Build history of the part. All positions in model axes, mm. A direction names the side the tool comes from. Round coordinates to 2 decimals unless told otherwise and drop trailing zeros. Loops run counter-clockwise (first coordinate to the right, second up) from the corner with the lowest first, then second, coordinate; pieces in that order, holes last. Notation, with made-up numbers: (-18, 11.25) - (16, 11.25) arc R36 cw to (16, 46.25) - close; hole circle Ø6 at (61, -35). An arc over 180 degrees is marked (long way). One line per question, with ' | ' between items. Start each with the question number.
from build123d import *

# Parameters (mm, degrees)
BOSS_EXTRUDE3_DEPTH = 11.049
SKETCH2_W           = 9.652
SKETCH2_H           = 6.604
SKETCH2_W_2         = 6.604
CUT_EXTRUDE1_DEPTH  = 8.255
SKETCH5_W           = 3.429
SKETCH5_H           = 5.08
BOSS_EXTRUDE4_DEPTH = 5.08
SKETCH6_W           = 9.652
SKETCH6_H           = 1.524
BOSS_EXTRUDE5_DEPTH = 5.08
CUT_EXTRUDE3_DEPTH  = 5.08
CUT_EXTRUDE4_START  = -0.0508
CUT_EXTRUDE4_DEPTH  = 0.0508
CUT_EXTRUDE5_DEPTH  = 0.0508


# Read off the part's stored shape, not the designer's step: Cut-Extrude4
with BuildPart() as part:
    # Sketch1 → Boss-Extrude3 (new body)
    with BuildSketch(Plane(origin=(0, 0, 0), x_dir=(1, 0, 0), z_dir=(0, 1, 0))):
        with BuildLine():
            ThreePointArc((-12.7635, 3.302), (-16.0655, 0), (-12.7635, -3.302))
            Line((-12.7635, -3.302), (-12.7635, -1.651))
            ThreePointArc((-12.7635, -1.651), (-14.4145, 0), (-12.7635, 1.651))
            Line((-12.7635, 1.651), (-12.7635, 3.302))
        make_face()
        with BuildLine():
            Line((-12.7635, -1.651), (-12.7635, -3.302))
            ThreePointArc((-12.7635, -3.302), (-10.428633409, -2.334866591), (-9.4615, 0))
            ThreePointArc((-9.4615, 0), (-10.428633409, 2.334866591), (-12.7635, 3.302))
            Line((-12.7635, 3.302), (-12.7635, 1.651))
            ThreePointArc((-12.7635, 1.651), (-11.596066704, 1.167433296), (-11.1125, 0))
            ThreePointArc((-11.1125, 0), (-11.596066704, -1.167433296), (-12.7635, -1.651))
        make_face()
        with BuildLine():
            Line((-12.7635, -3.302), (12.7635, -3.302))
            ThreePointArc((12.7635, -3.302), (9.4615, 0), (12.7635, 3.302))
            Line((12.7635, 3.302), (-12.7635, 3.302))
            ThreePointArc((-12.7635, 3.302), (-10.428633409, 2.334866591), (-9.4615, 0))
            ThreePointArc((-9.4615, 0), (-10.428633409, -2.334866591), (-12.7635, -3.302))
        make_face()
        with BuildLine():
            ThreePointArc((12.7635, 3.302), (9.4615, 0), (12.7635, -3.302))
            Line((12.7635, -3.302), (12.7635, -1.651))
            ThreePointArc((12.7635, -1.651), (11.1125, 0), (12.7635, 1.651))
            Line((12.7635, 1.651), (12.7635, 3.302))
        make_face()
        with BuildLine():
            Line((12.7635, -1.651), (12.7635, -3.302))
            ThreePointArc((12.7635, -3.302), (15.098366591, -2.334866591), (16.0655, 0))
            ThreePointArc((16.0655, 0), (15.098366591, 2.334866591), (12.7635, 3.302))
            Line((12.7635, 3.302), (12.7635, 1.651))
            ThreePointArc((12.7635, 1.651), (13.930933296, 1.167433296), (14.4145, 0))
            ThreePointArc((14.4145, 0), (13.930933296, -1.167433296), (12.7635, -1.651))
        make_face()
    extrude(amount=BOSS_EXTRUDE3_DEPTH)

    # Sketch2 → Cut-Extrude1 (cut)
    with BuildSketch(Plane(origin=(0, 11.049, 0), x_dir=(1, 0, 0), z_dir=(0, 1, 0))):
        Rectangle(SKETCH2_W, SKETCH2_H)
        with Locations((12.7635, 0)):
            Rectangle(SKETCH2_W_2, SKETCH2_H)
        with Locations((-12.7635, 0)):
            Rectangle(SKETCH2_W_2, SKETCH2_H)
    extrude(amount=-CUT_EXTRUDE1_DEPTH, mode=Mode.SUBTRACT)

    # Sketch5 → Boss-Extrude4 (add)
    with BuildSketch(Plane.XZ):
        with Locations((6.5405, 0.056957201)):
            Rectangle(SKETCH5_W, SKETCH5_H)
        with Locations((-6.5405, 0.056957201)):
            Rectangle(SKETCH5_W, SKETCH5_H)
    extrude(amount=BOSS_EXTRUDE4_DEPTH)

    # Sketch6 → Boss-Extrude5 (add)
    with BuildSketch(Plane.XZ):
        Rectangle(SKETCH6_W, SKETCH6_H)
    extrude(amount=BOSS_EXTRUDE5_DEPTH)

    # Sketch7 → Cut-Extrude3 (cut)
    with BuildSketch(Plane.XY.offset(0.762)):
        with BuildLine():
            ThreePointArc((-4.826, -5.08), (-0.756934481, -11.57255329), (5.052785714, -6.576785714))
            ThreePointArc((5.052785714, -6.576785714), (4.995767575, -5.819851233), (4.826, -5.08))
            Line((4.826, -5.08), (-4.826, -5.08))
        make_face()
        with BuildLine():
            Line((-4.826, -5.08), (4.826, -5.08))
            ThreePointArc((4.826, -5.08), (2.997307625, -2.50901108), (0, -1.524))
            ThreePointArc((0, -1.524), (-2.997307625, -2.50901108), (-4.826, -5.08))
        make_face()
    extrude(amount=-CUT_EXTRUDE3_DEPTH, mode=Mode.SUBTRACT)

    # Cut-Extrude4 outline → Cut-Extrude4 (cut)
    with BuildSketch(Plane(origin=(0, 11.049, 0), x_dir=(1, 0, 0), z_dir=(0, 1, 0)).offset(CUT_EXTRUDE4_START)):
        with BuildLine():
            Line((6.125651291, -1.107505234), (5.764715133, -1.322388012))
            add(Edge.make_bspline(
                [(5.764715133, -1.322388012), (5.795848726, -1.396544386), (5.855526361, -1.499286266), (5.978159662, -1.669974458), (6.05114933, -1.775594986), (6.148137968, -1.884253365), (6.256046735, -1.979672728), (6.372017343, -2.072531851), (6.478000588, -2.125037114), (6.583983834, -2.177542378), (6.687715089, -2.205891048), (6.772837481, -2.228601824), (6.855428053, -2.259126551), (6.956720766, -2.259126551), (7.082059087, -2.259126551), (7.202566961, -2.259126551), (7.355228923, -2.239958049), (7.545854824, -2.189191034), (7.64564176, -2.137070791), (7.756302185, -2.074391176), (7.861852333, -1.998233742), (7.956762183, -1.91923746), (8.138419792, -1.696975289), (8.222600111, -1.522442374), (8.284179667, -1.341062147), (8.308803358, -1.188392086), (8.308803358, -1.045195403), (8.257662319, -0.813306269), (8.216986985, -0.673773492), (8.132229192, -0.510521819), (7.993166094, -0.321750968), (7.909998502, -0.224416829), (7.802295587, -0.121226034), (7.6621337, 0.004412918), (7.5566666, 0.088832099), (7.079288797, 0.442114266), (6.827397054, 0.625925615), (6.758715893, 0.678132356), (6.698618911, 0.734864272), (6.648436244, 0.783693405), (6.615575385, 0.819143072), (6.575738864, 0.868399704), (6.535888686, 0.916871649), (6.495665853, 0.988895848), (6.455893708, 1.086814708), (6.435475968, 1.172671893), (6.422326559, 1.281945673), (6.441309585, 1.39829107), (6.467008859, 1.482949614), (6.517139065, 1.57939298), (6.576546974, 1.648262165), (6.660252521, 1.721257683), (6.76204807, 1.770361107), (6.850036001, 1.799422275), (6.919376094, 1.821827394), (7.000254698, 1.821827394), (7.060862271, 1.821827394), (7.158295762, 1.821827394), (7.245490979, 1.805342484), (7.330857485, 1.780448172), (7.394182968, 1.74575823), (7.422569964, 1.733524046), (7.454232705, 1.716179075), (7.490911825, 1.697072046), (7.514106284, 1.676478569), (7.564005826, 1.643675962), (7.656944095, 1.554409737), (7.739669602, 1.474435351), (7.776778642, 1.43169931), (7.842489762, 1.361666912), (7.905039475, 1.278267425)],
                knots=[0, 0, 0, 0, 0, 0, 0, 0, 0.015625, 0.03125, 0.046875, 0.0625, 0.078125, 0.09375, 0.109375, 0.125, 0.140625, 0.15625, 0.171875, 0.1875, 0.203125, 0.21875, 0.234375, 0.25, 0.265625, 0.28125, 0.296875, 0.3125, 0.328125, 0.34375, 0.359375, 0.375, 0.390625, 0.40625, 0.421875, 0.4375, 0.453125, 0.46875, 0.484375, 0.5, 0.515625, 0.53125, 0.546875, 0.5625, 0.578125, 0.59375, 0.609375, 0.625, 0.640625, 0.65625, 0.671875, 0.6875, 0.703125, 0.71875, 0.734375, 0.75, 0.765625, 0.78125, 0.796875, 0.8125, 0.828125, 0.84375, 0.859375, 0.875, 0.890625, 0.90625, 0.921875, 0.9375, 0.953125, 0.96875, 0.984375, 1, 1, 1, 1, 1, 1, 1, 1], degree=7))
            Line((7.905039475, 1.278267425), (8.253289165, 1.539455103))
            add(Edge.make_bspline(
                [(8.253289165, 1.539455103), (8.156895883, 1.66119447), (8.080596703, 1.752467641), (8.009921379, 1.822625174), (7.933726759, 1.919905891), (7.824588167, 2.017677373), (7.667478791, 2.113158926), (7.554717937, 2.174929753), (7.426668873, 2.21890102), (7.295363504, 2.247898039), (7.181818455, 2.267110724), (7.014103692, 2.267110724), (6.815864787, 2.237013824), (6.659136337, 2.182262131), (6.55037867, 2.129800369), (6.423181047, 2.050572345), (6.335021768, 1.976771869), (6.231051482, 1.855134106), (6.149145224, 1.716981286), (6.084448013, 1.567732126), (6.040533381, 1.421764923), (6.040533381, 1.293676397), (6.040533381, 1.143393573), (6.070495088, 0.985652762), (6.137396877, 0.821399612), (6.210558512, 0.692920171), (6.259072046, 0.646259485), (6.293158014, 0.580378426), (6.471822739, 0.420467618), (6.75149803, 0.193678775), (6.790287956, 0.170783169), (7.498283405, -0.384707414), (7.577864327, -0.459159137), (7.65987138, -0.544113603), (7.728973771, -0.621025877), (7.79510367, -0.718827072), (7.865584999, -0.866409444), (7.892864321, -0.947931981), (7.924722723, -1.016219237), (7.924722723, -1.066155835), (7.908904135, -1.168139886), (7.908904135, -1.225535848), (7.873403325, -1.31658975), (7.846091508, -1.386832441), (7.81374531, -1.446533535), (7.789405983, -1.495887306), (7.72836903, -1.555160993), (7.677947198, -1.604126212), (7.627570897, -1.65047546), (7.548458311, -1.699013274), (7.474880936, -1.729316994), (7.409037252, -1.764969223), (7.304160871, -1.794806682), (7.188897018, -1.818103802), (7.115683884, -1.818103802), (7.027185487, -1.818103802), (6.93589672, -1.818103802), (6.863229947, -1.796088084), (6.759400758, -1.765758188), (6.658680651, -1.706691455), (6.586423649, -1.661131989), (6.506706136, -1.594528182), (6.442547065, -1.533389449), (6.378433525, -1.469634745), (6.304296754, -1.382180872), (6.232995884, -1.281685995), (6.192311068, -1.220896958), (6.149245652, -1.146989207), (6.125651291, -1.107505234)],
                knots=[0, 0, 0, 0, 0, 0, 0, 0, 0.016129032, 0.032258065, 0.048387097, 0.064516129, 0.080645161, 0.096774194, 0.112903226, 0.129032258, 0.14516129, 0.161290323, 0.177419355, 0.193548387, 0.209677419, 0.225806452, 0.241935484, 0.258064516, 0.274193548, 0.290322581, 0.306451613, 0.322580645, 0.338709677, 0.35483871, 0.370967742, 0.387096774, 0.403225806, 0.419354839, 0.435483871, 0.451612903, 0.467741935, 0.483870968, 0.5, 0.516129032, 0.532258065, 0.548387097, 0.564516129, 0.580645161, 0.596774194, 0.612903226, 0.629032258, 0.64516129, 0.661290323, 0.677419355, 0.693548387, 0.709677419, 0.725806452, 0.741935484, 0.758064516, 0.774193548, 0.790322581, 0.806451613, 0.822580645, 0.838709677, 0.85483871, 0.870967742, 0.887096774, 0.903225806, 0.919354839, 0.935483871, 0.951612903, 0.967741935, 0.983870968, 1, 1, 1, 1, 1, 1, 1, 1], degree=7))
        make_face()
    extrude(amount=CUT_EXTRUDE4_DEPTH, mode=Mode.SUBTRACT)

    # Sketch10 → Cut-Extrude5 (cut)
    with BuildSketch(Plane(origin=(0, 11.049, 0), x_dir=(1, 0, 0), z_dir=(0, 1, 0))):
        Polygon((-5.758009801, 2.155020867), (-5.758009801, 1.720550301), (-7.809265142, 1.720550301), (-7.809265142, 0.395375626), (-5.758009801, 0.395375626), (-5.758009801, -0.057812947), (-7.809265142, -0.057812947), (-7.809265142, -1.718355868), (-5.758009801, -1.718355868), (-5.758009801, -2.159), (-8.188893002, -2.159), (-8.188893002, 2.155020867), align=None)
    extrude(amount=-CUT_EXTRUDE5_DEPTH, mode=Mode.SUBTRACT)


solid = part.part
1) Saw through at C-C on x = -14. Write the cut outline in (y, z), and give its area (3 significant figures).
2) Drop flat-ended pins along their axis: pin 1 (2 mm diameter, centred on x = -12.5, z = -1.5, fed in from +Y); pin 2 (2.5 mm diameter, centred on x = -7.5, y = -1.5, fed in from +Z); pin 3 (0.6 mm diameter, centred on y = -3, z = 2, fed in from +X) (3 decimals). Give the stop position or say it passes through.
3) Tool access for faces 5 (the flat face through (-7, -3, -2.483)), 6 (the flat face through (-12, 2.794, -2)), 7 (the flat face through (7.4, 10.998, 0)), 8 (the flat face through (-7, -3, 2.597)): list every direction of +Z, -Z, +X, -X, +Y, -Y with a clear straight run to the whole face (end or side of a thin tool).
4) Wall check: line 1 (X direction, y = 5.75, z = -3); line 2 (X direction, y = -3.75, z = 2.5) (3 decimals); line 3 (Y direction, x = -1, z = 2.25). Give the ranges that are in metal, low to high. Write a range as [from, to].
5) Saw through at D-D on y = -3.5. Write the cut outline in (x, z) (3 decimals).
6) Two-plate mould, pull along X, no slides. Class faces 1 (the flat face through (-4.826, 7, 0)), 2 (the flat face through (9.462, 7, 0)), 3 (the flat face through (0, -1, 0.762)), 4 (the flat face through (0, 2, -3.302)): +X half, -X half, draft (parallel to the pull), parting line (faces both ways), or undercut.
7) Saw through at A-A on y = 5. Write the cut outline in (x, z), and give its area (3 significant figures).
8) Saw through at B-B on y = 2.5. Write the cut outline in (x, z).
Answer key:
1) outline: (0, -3.06) - (2.79, -3.06) - (2.79, -1.09) - (0, -1.09) - close; (0, 1.09) - (2.79, 1.09) - (2.79, 3.06) - (0, 3.06) - close | area: 11.0 mm²
2) pin 1: y = 2.79 | pin 2: z = 2.6 | pin 3: x = 8.255
3) face 5: -Z, +X, -X, -Y | face 6: +Z, -Z, -X, +Y | face 7: +Y | face 8: +Z, +X, -X, -Y
4) line 1: [-9.46, -4.83], [4.83, 9.46] | line 2: [-8.255, -4.826], [4.826, 8.255] | line 3: [0, 2.79]
5) outline: (-8.255, -2.483) - (-4.826, -2.483) - (-4.826, -0.762) - (-4.008, -0.762) - (-4.008, 0.762) - (-4.826, 0.762) - (-4.826, 2.597) - (-8.255, 2.597) - close; (4.008, -0.762) - (4.826, -0.762) - (4.826, -2.483) - (8.255, -2.483) - (8.255, 2.597) - (4.826, 2.597) - (4.826, 0.762) - (4.008, 0.762) - close
6) face 1: undercut | face 2: +X half | face 3: undercut | face 4: draft
7) outline: (-9.46, -3.3) - (-4.83, -3.3) - (-4.83, 3.3) - (-9.46, 3.3) - close; (4.83, -3.3) - (9.46, -3.3) - (9.46, 3.3) - (4.83, 3.3) - close | area: 61.2 mm²
8) outline: (-12.76, -3.3) - (12.76, -3.3) arc R3.3 ccw to (12.76, 3.3) - (-12.76, 3.3) arc R3.3 ccw to start; hole circle Ø3.3 at (-12.76, 0); hole circle Ø3.3 at (12.76, 0)
